Check sheet for the drawn part. Datum: minimum x, y, z corner. Units: mm. Give positions to 0.01 mm unless a question says otherwise; leave off trailing zeros. Loops run counter-clockwise (first coordinate to the right, second up) from the corner with the lowest first, then second, coordinate; pieces in that order, holes last. Notation, with made-up numbers: (54.5, 6) - (64.5, 6) arc R20 cw to (64.5, 29) - close; hole circle Ø3 at (-27, -17). An arc over 180 degrees is marked (long way). Answer in a Markdown table with one row per item.
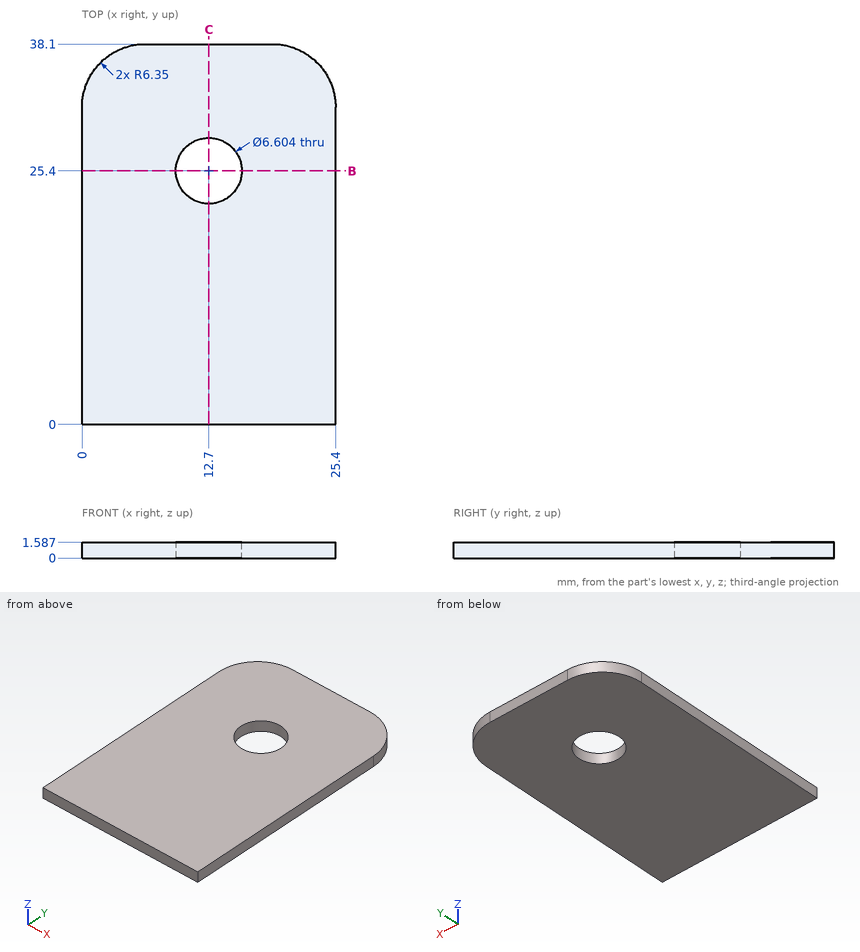
Q1. Thickness scan on line 1 (X direction, y = 25.4, z = 0.45); line 2 (Y direction, x = 12.7, z = 0.4); line 3 (Y direction, x = 10.75, z = 1.15) (1 decimal). Record the ranges inside material, lowest first.
Completed:
| item | result |
|---|---|
| line 1 | 0 to 9.4, 16 to 25.4 |
| line 2 | 0 to 22.1, 28.7 to 38.1 |
| line 3 | 0 to 22.7, 28.1 to 38.1 |
Q2. Sectioned sample at C-C (x = 12.7). Record the cut outline in (y, z).
Completed:
| item | result |
|---|---|
| outline | (0, 0) - (22.1, 0) - (22.1, 1.59) - (0, 1.59) - close; (28.7, 0) - (38.1, 0) - (38.1, 1.59) - (28.7, 1.59) - close |
Q3. Sectioned sample at B-B (y = 25.4). Record the cut outline in (x, z).
Completed:
| item | result |
|---|---|
| outline | (0, 0) - (9.4, 0) - (9.4, 1.59) - (0, 1.59) - close; (16, 0) - (25.4, 0) - (25.4, 1.59) - (16, 1.59) - close |
